Here's the drawing with two shaded views (mm, measured from the low corner). I have some questions. Give positions to 0.01 mm unless a question says otherwise; leave off trailing zeros. Loops run counter-clockwise (first coordinate to the right, second up) from the corner with the lowest first, then second, coordinate; pieces in that order, holes last. Notation, with made-up numbers: (17, -3.75) - (62, -3.75) arc R24 ccw to (62, 31.25) - close; hole circle Ø9 at (14, 70.25). An arc over 180 degrees is marked (long way). Use a Markdown table: item, result. Add a question column.
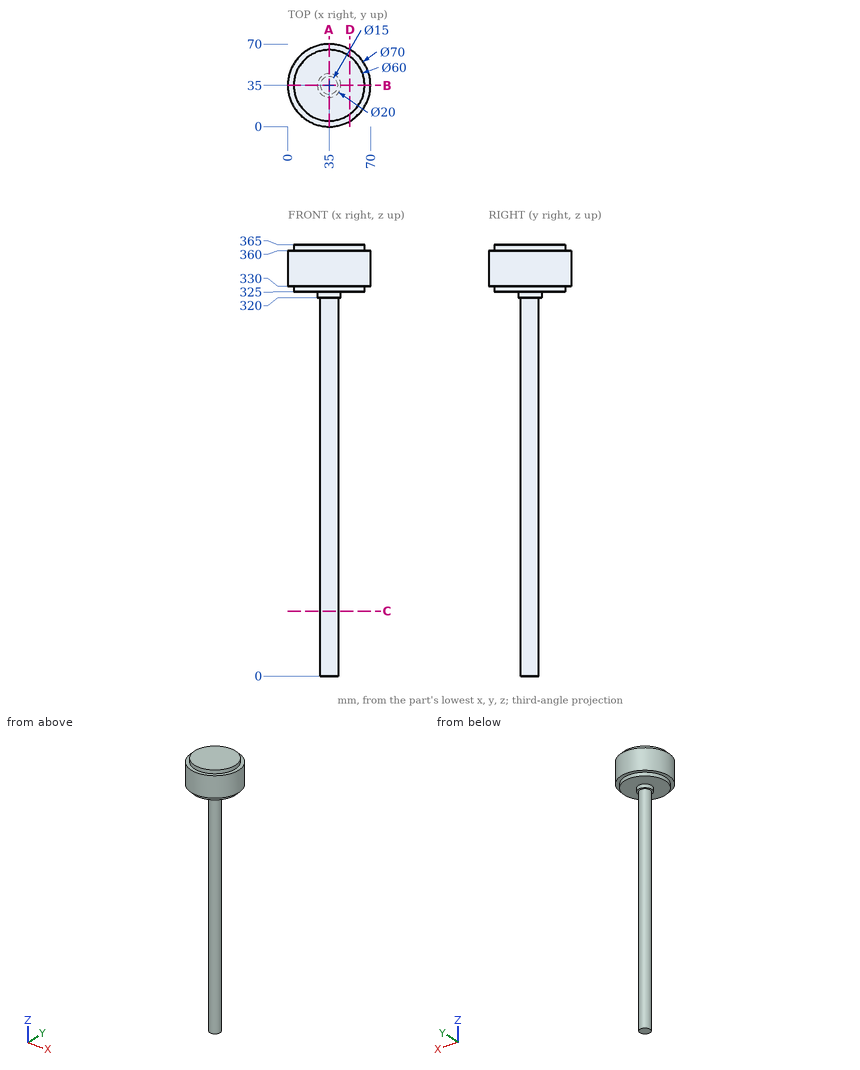
1. Suppose I cut it at C-C (z = 55). List the corners of the cut face in (x, y) for me, and give its area (3 significant figures).
2. Suppose I cut it at A-A (x = 35). List the corners of the cut face in (y, z) for me, and give its area (3 significant figures).
3. Suppose I cut it at D-D (x = 52.5). List the corners of the cut face in (y, z) for me, and give its area (3 significant figures).
4. Will these pins go through, and if not, where does the flat tip stop? P1, Ø6, axis at x = 36, y = 37, coming from the -Z side; P2, Ø5, axis at x = 27, y = 56.5, coming from the -Z side; P3, Ø6, axis at y = 43.5, z = 240.5, coming from the -X side; P4, Ø6, axis at x = 39, z = 39, coming from the -Y side.
5. Please list where these lines run through material, in increasing order: line 1 along Z through (x, y) = (9, 49.5); line 2 along Y through (x, z) = (35, 108.5); line 3 along Z through (x, y) = (55, 9). Write a range as [from, to].
Results below:
| question | item | result |
|---|---|---|
| 1 | outline | circle Ø15 at (35, 35) |
| 1 | area | 177 mm² |
| 2 | outline | (0, 330) - (5, 330) - (5, 325) - (25, 325) - (25, 320) - (27.5, 320) - (27.5, 0) - (42.5, 0) - (42.5, 320) - (45, 320) - (45, 325) - (65, 325) - (65, 330) - (70, 330) - (70, 360) - (65, 360) - (65, 365) - (5, 365) - (5, 360) - (0, 360) - close |
| 2 | area | 7,600 mm² |
| 3 | outline | (4.69, 330) - (10.63, 330) - (10.63, 325) - (59.37, 325) - (59.37, 330) - (65.31, 330) - (65.31, 360) - (59.37, 360) - (59.37, 365) - (10.63, 365) - (10.63, 360) - (4.69, 360) - close |
| 3 | area | 2,310 mm² |
| 4 | P1 | z = 0 |
| 4 | P2 | z = 325 |
| 4 | P3 | x = 29.9 |
| 4 | P4 | y = 27.57 |
| 5 | line 1 | [325, 365] |
| 5 | line 2 | [27.5, 42.5] |
| 5 | line 3 | [330, 360] |
